Input: part model. Units: mm. Frame: model coordinates. A direction names the side the tool comes from. Coordinates: 2 decimals unless noted, no trailing zeros. Write each loop counter-clockwise with the first axis right and the second up, starting at its lowest first coordinate (ties: lowest second). Pieces come first, ordered by that corner, then holes.
from build123d import *

# Parameters (mm, degrees)
SKETCH1_R           = 12.573
SKETCH1_R_2         = 5.715
BOSS_EXTRUDE1_DEPTH = 25.4
CUT_EXTRUDE2_START  = -6.35
SKETCH3_R           = 6.35
SKETCH3_R_2         = 5.715
CUT_EXTRUDE2_DEPTH  = 6.35
SKETCH4_R           = 6.35
SKETCH4_R_2         = 5.715
CUT_EXTRUDE3_DEPTH  = 6.35


with BuildPart() as part:
    # Sketch1 → Boss-Extrude1 (new body)
    with BuildSketch(Plane(origin=(0, 0, 0), x_dir=(1, 0, 0), z_dir=(0, 1, 0))):
        with Locations(Location((0, 0, 0), (0, 0, 270))):
            Circle(SKETCH1_R)
        with Locations(Location((0, 0, 0), (0, 0, 270))):
            Circle(SKETCH1_R_2, mode=Mode.SUBTRACT)
    extrude(amount=BOSS_EXTRUDE1_DEPTH)

    # Sketch3 → Cut-Extrude2 (cut)
    with BuildSketch(Plane(origin=(0, 25.4, 0), x_dir=(1, 0, 0), z_dir=(0, 1, 0)).offset(CUT_EXTRUDE2_START)):
        with Locations(Location((0, 0, 0), (0, 0, 270))):
            Circle(SKETCH3_R)
        with Locations(Location((0, 0, 0), (0, 0, 270))):
            Circle(SKETCH3_R_2, mode=Mode.SUBTRACT)
    extrude(amount=CUT_EXTRUDE2_DEPTH, mode=Mode.SUBTRACT)

    # Sketch4 → Cut-Extrude3 (cut)
    with BuildSketch(Plane.XZ):
        with Locations(Location((0, 0, 0), (0, 0, 90))):
            Circle(SKETCH4_R)
        with Locations(Location((0, 0, 0), (0, 0, 270))):
            Circle(SKETCH4_R_2, mode=Mode.SUBTRACT)
    extrude(amount=-CUT_EXTRUDE3_DEPTH, mode=Mode.SUBTRACT)


solid = part.part
Item 1: Section query D-D, the plane x = -8.25. Return loops of the section in (y, z).
Item 2: Section query B-B, the plane z = 0. Return loops of the section in (x, y) (3 decimals), then the cut area to 3 significant figures.
Item 3: Material intervals for line 1 (X direction, y = 2.25, z = 0); line 2 (X direction, y = 13.5, z = 0) (3 decimals); line 3 (Z direction, x = -0.75, y = 19.25), sorted ascending.
Item 4: Section query A-A, the plane x = 0. Return loops of the section in (y, z) (3 decimals), then the cut area to 3 significant figures.
Item 5: Pull-direction query (Z, two-part tool) for faces 1 (the face through (1, 19.05, -6)), 2 (the face through (-12.274, 12.522, -2.726)), 3 (the face through (3, 0, -6)); classes: released by +Z, released by -Z, zero draft, split by the parting line, or undercut.
Item 6: Pin query (flat end, axial travel): pin 1 Ø6.5 at (x, z) = (-1.5, 2) entering from +Y; pin 2 Ø7 at (x, z) = (0, 0) entering from -Y; pin 3 Ø12 at (x, y) = (7, 14) entering from -Z; pin 4 Ø1 at (y, z) = (12, 1) entering from -X. Return the tip coordinate at first contact, or that it passes through.
Item 7: Access query for faces 4 (the face through (3, 25.4, -6)), 5 (the face through (3.86, 3.13, -5.04)), 6 (the face through (-3.86, 22.18, -5.04)). Directions: +Z, -Z, +X, -X, +Y, -Y. A direction counts if a zero-diameter tool reaches every point of the face in a straight line with its end or side. Return the directions, or none.
Item 8: Section query C-C, the plane y = 8. Return loops of the section in (x, z) (3 decimals).
The answers:
1. outline: (0, -9.49) - (25.4, -9.49) - (25.4, 9.49) - (0, 9.49) - close
2. outline: (-12.573, 0) - (-6.35, 0) - (-6.35, 6.35) - (-5.715, 6.35) - (-5.715, 19.05) - (-6.35, 19.05) - (-6.35, 25.4) - (-12.573, 25.4) - close; (5.715, 6.35) - (6.35, 6.35) - (6.35, 0) - (12.573, 0) - (12.573, 25.4) - (6.35, 25.4) - (6.35, 19.05) - (5.715, 19.05) - close
2. area: 332 mm2
3. line 1: x = -12.57 to -6.35, 6.35 to 12.57
3. line 2: x = -12.573 to -5.715, 5.715 to 12.573
3. line 3: z = -12.55 to -6.31, 6.31 to 12.55
4. outline: (0, -12.573) - (25.4, -12.573) - (25.4, -6.35) - (19.05, -6.35) - (19.05, -5.715) - (6.35, -5.715) - (6.35, -6.35) - (0, -6.35) - close; (0, 6.35) - (6.35, 6.35) - (6.35, 5.715) - (19.05, 5.715) - (19.05, 6.35) - (25.4, 6.35) - (25.4, 12.573) - (0, 12.573) - close
4. area: 332 mm2
5. face 1: undercut
5. face 2: split by the parting line
5. face 3: zero draft
6. pin 1: stops at y = 19.05
6. pin 2: passes through
6. pin 3: stops at z = -12.53
6. pin 4: stops at x = -12.56
7. face 4: +Z, -Z, +X, -X, +Y
7. face 5: -Y
7. face 6: +Y
8. outline: circle Ø25.146 at (0, 0); hole circle Ø11.43 at (0, 0)
